Check sheet for the modelled part. Datum: model origin and axes. Units: mm. A direction names the side the tool comes from. Coordinates: 2 decimals unless noted, no trailing zeros. Write each loop counter-clockwise with the first axis right and the second up, starting at its lowest first coordinate (ties: lowest second). Pieces come first, ordered by that corner, then holes. Notation, with made-up numbers: (-3.75, -5.5) - (17.25, -5.5) arc R30 ccw to (17.25, 19.5) - close; hole circle Ø1 at (-21.75, 5.5). An arc over 180 degrees is marked (long way). Use one line per item in the form item = value. Start each with the question number.
1. Tool access check on faces 1 (the face through (28, 2, 0)), 2 (the face through (-117.15, -11.02, 13.5)), 3 (the face through (35.43, 56, 14)), 4 (the face through (0, 51.345, 14)), 5 (the face through (-46.35, 22.83, 13.5)). Record the directions out of +Z, -Z, +X, -X, +Y, -Y that give a thin tool (end or side, any length) a straight path to the whole face; none if there is none.
2. Draft check along Y on faces 6 (the face through (0, 57, 19.812)), 7 (the face through (-35.261, 4, 14)), 8 (the face through (0, -53.473, 14)). Enter one of: +Y half, -Y half, draft (parallel to the pull), parting line (faces both ways), or undercut.
3. Cross-section at A-A on z = 16.75. Give the number of separate pieces and of enclosed holes in the cut face, then the cut area to 3 significant figures.
4. Cross-section at B-B on x = 75. Record the boundary of the cut face in (y, z), then the cut area to 3 significant figures.
5. Scan lines: line 1 along Z through (x, y) = (57.5, -40); line 2 along Y through (x, z) = (-82, 15.75); line 3 along X through (y, z) = (-42, 16.75). Record each from-to range of solid material in increasing order.
6. Go/stop test with flat-tipped pins: pin 1 Ø1.9 at (y, z) = (7.5, 14) entering from -X; pin 2 Ø6 at (x, z) = (9, 11.5) entering from +Y; pin 3 Ø2.5 at (x, z) = (214, 15.5) entering from -Y. Record where each tip stops, or that it passes through.
```python
from build123d import *

# Parameters (mm, degrees)
F0_W     = 468.000487
F0_H     = 137.646742
F1_DEPTH = 7.366
F2_W     = 70.247736
F2_H     = 10.415282
F2_W_2   = 70.469331
F2_H_2   = 11.744887
F2_H_3   = 11.301685
F2_W_3   = 70.91254
F2_H_4   = 13.074499
F3_DEPTH = 12.446


with BuildPart() as f1:
    # F0 (on Top) → F1 (new body)
    with BuildSketch(Plane.XY):
        with Locations((31.531855, 0.796761)):
            Rectangle(F0_W, F0_H)
    extrude(amount=F1_DEPTH)

    # F2 (on face) → F3 (join)
    with BuildSketch(Plane.XY.offset(7.366)):
        Polygon((-138.646447, 5.454973), (-156.350389, 5.454973), (-202.468388, 5.454973), (-202.468388, 1.403027), (-156.604389, 1.403027), (-138.416419, 1.403027), (-95.286213, -23.789594), (-59.45519, -23.789594), (-37.736211, -36.710622), (0, -36.710622), (37.736211, -36.710622), (59.45519, -23.789594), (95.286213, -23.789594), (138.416419, 1.403027), (156.604389, 1.403027), (181.72892, 1.403027), (183.610221, 1.405067), (183.59076, -2.286332), (186.661547, -2.286332), (186.661547, 1.475384), (189.655577, 1.475384), (189.655577, -2.286332), (192.649593, -2.286332), (192.649593, 1.475384), (195.873921, 1.475384), (195.873921, -2.286332), (199.09825, -2.286332), (199.09825, 1.475384), (202.476119, 1.475384), (202.476119, -2.286332), (206.237828, -2.286332), (206.237828, 1.475384), (209.615698, 1.475384), (209.615698, -2.286332), (213.147109, -2.286332), (213.147109, 1.475384), (216.14114, 1.475384), (216.14114, -2.286332), (219.135156, -2.286332), (219.135156, 1.475384), (222.359484, 1.475384), (222.359484, -2.286332), (225.583812, -2.286332), (225.583812, 1.475384), (228.961682, 1.475384), (228.961682, -2.286332), (232.72339, -2.286332), (232.72339, 1.475384), (236.10126, 1.475384), (236.10126, -2.286332), (239.886671, -2.286332), (239.886671, 1.519807), (265.532099, 1.473806), (265.532099, 5.592193), (239.886671, 5.592193), (239.886671, 9.353909), (236.35526, 9.353909), (236.35526, 5.592193), (232.97739, 5.592193), (232.97739, 9.353909), (229.215682, 9.353909), (229.215682, 5.592193), (225.837812, 5.592193), (225.837812, 9.353909), (222.613484, 9.353909), (222.613484, 5.592193), (219.389156, 5.592193), (219.389156, 9.353909), (216.39514, 9.353909), (216.39514, 5.592193), (213.401109, 5.592193), (213.401109, 9.353909), (209.869698, 9.353909), (209.869698, 5.592193), (206.491828, 5.592193), (206.491828, 9.353909), (202.730119, 9.353909), (202.730119, 5.592193), (199.35225, 5.592193), (199.35225, 9.353909), (196.127921, 9.353909), (196.127921, 5.592193), (192.903593, 5.592193), (192.903593, 9.353909), (189.909577, 9.353909), (189.909577, 5.592193), (186.915547, 5.592193), (186.915547, 9.353909), (183.864221, 9.353909), (183.864221, 5.446596), (181.752861, 5.454973), (156.350389, 5.454973), (138.646447, 5.454973), (95.279287, 33.300258), (57.058044, 33.300258), (35.339065, 45.953158), (0, 45.953158), (-35.339065, 45.953158), (-57.058044, 33.300258), (-95.279287, 33.300258), align=None)
        Polygon((-37.810078, -32.348648), (-55.936935, -21.585828), (-37.810078, -10.823006), (0, -10.823006), (37.810078, -10.823006), (55.936935, -21.585828), (37.810078, -32.348648), (0, -32.348648), align=None, mode=Mode.SUBTRACT)
        Polygon((-135.340132, 3.482032), (-95.286213, 29.199943), (-57.058044, 29.199943), (-35.339065, 16.278915), (0, 16.278915), (35.339065, 16.278915), (57.058044, 29.199943), (95.286213, 29.199943), (135.340132, 3.482032), (95.286213, -19.91371), (59.45519, -19.91371), (37.736211, -7.260809), (0, -7.260809), (-37.736211, -7.260809), (-59.45519, -19.91371), (-95.286213, -19.91371), align=None, mode=Mode.SUBTRACT)
        Polygon((-35.358623, 20.574907), (-53.485479, 31.337727), (-35.358623, 42.100549), (0, 42.100549), (35.358623, 42.100549), (53.485479, 31.337727), (35.358623, 20.574907), (0, 20.574907), align=None, mode=Mode.SUBTRACT)
        with Locations((0.305964, 56.552144)):
            Rectangle(F2_W, F2_H)
        with Locations((0.416769, -47.60065)):
            Rectangle(F2_W_2, F2_H_2)
        with Locations((0.259081, 31.408699)):
            Rectangle(F2_W, F2_H_3)
        with Locations((0.195164, 4.475746)):
            Rectangle(F2_W_3, F2_H_4)
        with Locations((0.247676, -21.536928)):
            Rectangle(F2_W, F2_H_3)
    extrude(amount=F3_DEPTH)


solid = f1.part
```
Final values:
q1.face_1 = -Z, +X, -X, +Y, -Y
q1.face_2 = +Z, -X, -Y
q1.face_3 = +Z, +X, +Y
q1.face_4 = +Z, +X, -X
q1.face_5 = +Z
q2.face_6 = draft
q2.face_7 = undercut
q2.face_8 = -Y half
q3.separate_pieces = 6
q3.enclosed_holes = 3
q3.area = 8,200 mm²
q4.outline = (-68.03, 0) - (69.62, 0) - (69.62, 7.37) - (33.3, 7.37) - (33.3, 19.81) - (29.2, 19.81) - (29.2, 7.37) - (-19.91, 7.37) - (-19.91, 19.81) - (-23.79, 19.81) - (-23.79, 7.37) - (-68.03, 7.37) - close
q4.area = 1,110 mm²
q5.line_1 = 0 to 7.37
q5.line_2 = -23.79 to -19.91, 29.2 to 33.3
q5.line_3 = -34.82 to 35.65
q6.pin_1 = -136.94
q6.pin_2 = 61.76
q6.pin_3 = -2.29
